Geometry: see drawing. Coordinates: mm, zero at the bounding-box minimum. Give positions to 0.01 mm unless a question says otherwise; leave off trailing zeros. Loops run counter-clockwise (first coordinate to the right, second up) from the corner with the lowest first, then second, coordinate; pieces in that order, holes last. Notation, with made-up numbers: (49, 18.25) -> (57, 18.25) arc R7 cw to (57, 25.25) -> close; hole circle Ø7 at (-1.5, 81). An arc over 180 degrees is marked (long way). Use CSV: the item, a comma, the result in double quotes.
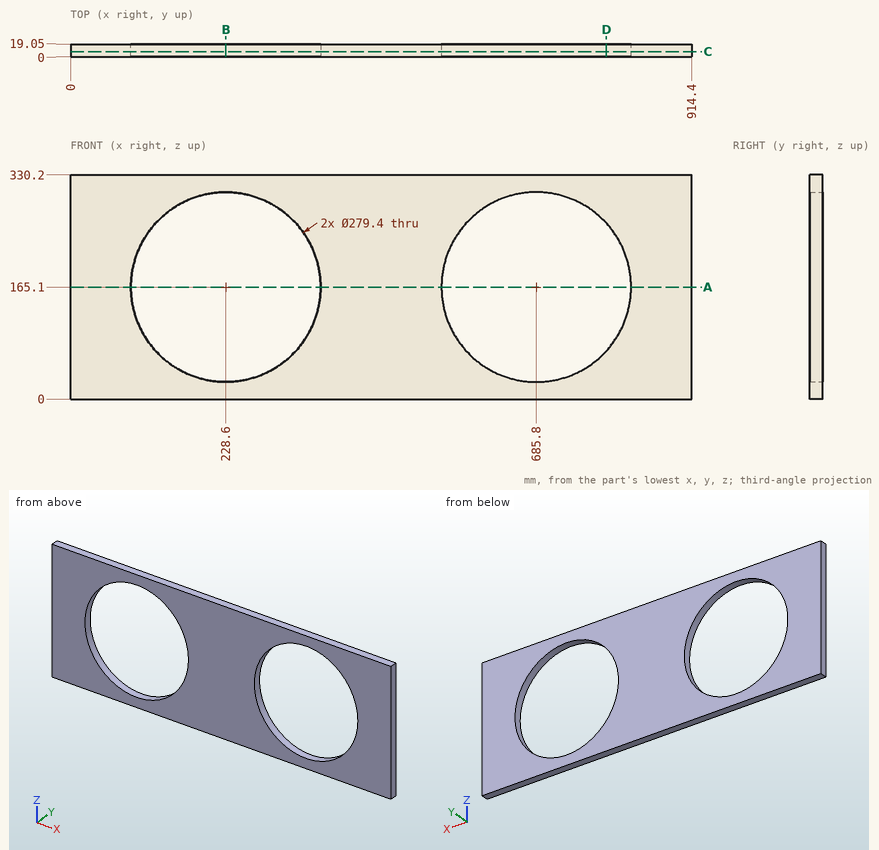
1) Section query B-B (x = 228.6). Return loops of the section in (y, z), then the cut area to 3 significant figures.
From the geometry:
outline,"(0, 0) -> (19.05, 0) -> (19.05, 25.4) -> (0, 25.4) -> close; (0, 304.8) -> (19.05, 304.8) -> (19.05, 330.2) -> (0, 330.2) -> close"
area,"968 mm^2"
2) Section query A-A (z = 165.1). Return loops of the section in (x, y), then the cut area to 3 significant figures.
From the geometry:
outline,"(0, 0) -> (88.9, 0) -> (88.9, 19.05) -> (0, 19.05) -> close; (368.3, 0) -> (546.1, 0) -> (546.1, 19.05) -> (368.3, 19.05) -> close; (825.5, 0) -> (914.4, 0) -> (914.4, 19.05) -> (825.5, 19.05) -> close"
area,"6,770 mm^2"
3) Section query C-C (y = 8). Return loops of the section in (x, z), then the cut area to 3 significant figures.
From the geometry:
outline,"(0, 0) -> (914.4, 0) -> (914.4, 330.2) -> (0, 330.2) -> close; hole circle Ø279.4 at (228.6, 165.1); hole circle Ø279.4 at (685.8, 165.1)"
area,"179,000 mm^2"
4) Section query D-D (x = 789). Return loops of the section in (y, z).
From the geometry:
outline,"(0, 0) -> (19.05, 0) -> (19.05, 70.94) -> (0, 70.94) -> close; (0, 259.26) -> (19.05, 259.26) -> (19.05, 330.2) -> (0, 330.2) -> close"
5) Ray query, line 1 (Z direction, x = 685.8, y = 13.75); line 2 (X direction, y = 2.75, z = 87.5); line 3 (X direction, y = 9, z = 61). Return the intervals inside material, ascending.
From the geometry:
line 1,"z = 0 to 25.4, 304.8 to 330.2"
line 2,"x = 0 to 112.43, 344.77 to 569.63, 801.97 to 914.4"
line 3,"x = 0 to 135.44, 321.76 to 592.64, 778.96 to 914.4"
